```python
from build123d import *

# Parameters (mm, degrees)
SKETCH1_R           = 2.5
BOSS_EXTRUDE1_DEPTH = 24
BOSS_EXTRUDE2_START = -5
SKETCH2_R           = 10
BOSS_EXTRUDE2_DEPTH = 14


with BuildPart() as part:
    # Sketch1 → Boss-Extrude1 (new body)
    with BuildSketch(Plane.XY):
        Circle(SKETCH1_R)
    extrude(amount=BOSS_EXTRUDE1_DEPTH)

    # Sketch2 → Boss-Extrude2 (add)
    with BuildSketch(Plane.XY.offset(24).offset(BOSS_EXTRUDE2_START)):
        Circle(SKETCH2_R)
    extrude(amount=-BOSS_EXTRUDE2_DEPTH)


solid = part.part
```
CAD build for the part. Positions are in the model's coordinates, mm. A direction names the side the tool comes from. Coordinates: 2 decimals unless noted, no trailing zeros. Write each loop counter-clockwise with the first axis right and the second up, starting at its lowest first coordinate (ties: lowest second). Pieces come first, ordered by that corner, then holes. Notation, with made-up numbers: (-3.75, -16) -> (9.25, -16) arc R8 ccw to (9.25, -10) -> close; hole circle Ø9 at (-16.75, 12.5). An arc over 180 degrees is marked (long way). Return JSON: item names as keys, results as strings. Group by question number.
Q1. Drill centre lines: line 1 (Z direction, x = 1.5, y = -5); line 2 (Y direction, x = 1.75, z = 9); line 3 (X direction, y = 0.75, z = 16). Where is each one in solid material? Low to high.
Q2. Cut at A-A, the plane y = 0. Give the cut face in (x, z), then the cut area to 3 significant figures.
Q3. Cut at D-D, the plane y = -4.25. Give the cut face in (x, z).
Q4. Which spindle directions (+Z, -Z, +X, -X, +Y, -Y) get a long thin tool onto all of the face, cutting with end or side? Do faces 1 (the face through (-0.54, -2.44, 21.46)), 2 (the face through (2, -2, 5)), 3 (the face through (0, 0, 0)). Say none if no direction does.
Q5. Flat gauge pins, fed straight in: pin 1 (5 mm diameter, centred on x = 6, z = 7.5, fed in from +Y); pin 2 (2 mm diameter, centred on x = -0.5, y = -6, fed in from -Z); pin 3 (8 mm diameter, centred on y = -6, z = 12.5, fed in from -X); pin 4 (12 mm diameter, centred on x = -6, y = 2.5, fed in from +Z). Where does each tip first touch, or does it go through?
Q6. Cut at C-C, the plane z = 3.5. Give the cut face in (x, y), then the cut area to 3 significant figures.
Returned:
{
 "1": {"line 1": "z = 5 to 19", "line 2": "y = -9.85 to 9.85", "line 3": "x = -9.97 to 9.97"},
 "2": {"outline": "(-10, 5) -> (-2.5, 5) -> (-2.5, 0) -> (2.5, 0) -> (2.5, 5) -> (10, 5) -> (10, 19) -> (2.5, 19) -> (2.5, 24) -> (-2.5, 24) -> (-2.5, 19) -> (-10, 19) -> close", "area": "330 mm2"},
 "3": {"outline": "(-9.05, 5) -> (9.05, 5) -> (9.05, 19) -> (-9.05, 19) -> close"},
 "4": {"face 1": "+Z", "face 2": "-Z", "face 3": "-Z, +X, -X, +Y, -Y"},
 "5": {"pin 1": "stops at y = 9.37", "pin 2": "stops at z = 5", "pin 3": "stops at x = -9.8", "pin 4": "stops at z = 24"},
 "6": {"outline": "circle Ø5 at (0, 0)", "area": "19.6 mm2"}
}
